from build123d import *

# Parameters (mm, degrees)
EXTRUDE_1_DEPTH     = 360
CUT_EXTRUDE_1_DEPTH = 702.498396292


with BuildPart() as part:
    # 草图1 → 凸台-拉伸1 (new body)
    with BuildSketch(Plane(origin=(0, 0, 0), x_dir=(1, 0, 0), z_dir=(0, 1, 0))):
        Polygon((-225, 0), (225, 0), (225, 250), (100, 400), (-100, 400), (-225, 250), align=None)
    extrude(amount=EXTRUDE_1_DEPTH)

    # 草图2 → 切除-拉伸1 (cut, through all)
    with BuildSketch(Plane(origin=(225, 0, 0), x_dir=(0, 0, -1), z_dir=(1, 0, 0))):
        Polygon((250, 360), (400, 227.712434447), (400, 360), align=None)
    extrude(amount=-CUT_EXTRUDE_1_DEPTH, mode=Mode.SUBTRACT)


solid = part.part
Part model, mm, in its own coordinate system. Give positions to 0.01 mm unless a question says otherwise; leave off trailing zeros. Write each loop counter-clockwise with the first axis right and the second up, starting at its lowest first coordinate (ties: lowest second). Pieces come first, ordered by that corner, then holes.
1) Probe L1, parallel to Z at x = 101, y = 100.5; L2, parallel to Z at x = 22.5, y = 232.5; L3, parallel to Y at x = 62, z = -251. List the from-to ranges inside material, lowest first.
Resolved:
L1: z = -398.8 to 0
L2: z = -394.57 to 0
L3: y = 0 to 359.12
2) Cut at B-B on y = 92. Write the cut outline in (x, z), then the cut area to 3 significant figures.
Resolved:
outline: (-225, -250) - (-100, -400) - (100, -400) - (225, -250) - (225, 0) - (-225, 0) - close
area: 161,000 mm2
3) Cut at A-A on x = 27.5. Write the cut outline in (y, z).
Resolved:
outline: (0, -400) - (227.71, -400) - (360, -250) - (360, 0) - (0, 0) - close
4) Cut at C-C on z = -357. Write the cut outline in (x, y), then the cut area to 3 significant figures.
Resolved:
outline: (-135.83, 0) - (135.83, 0) - (135.83, 265.63) - (-135.83, 265.63) - close
area: 72,200 mm2
5) Pin check, flat tips, straight feed: pin 1 (1 mm diameter, centred on y = 164.5, z = -345.5, fed in from +X); pin 2 (4 mm diameter, centred on y = 284.5, z = -324.5, fed in from -X); pin 3 (1.5 mm diameter, centred on y = 288, z = -264, fed in from -X). Stop position of each tip, or through.
Resolved:
pin 1: stops at x = 145.83
pin 2: stops at x = -164.58
pin 3: stops at x = -213.96
6) Cut at D-D on x = 132. Write the cut outline in (y, z).
Resolved:
outline: (0, -361.6) - (261.58, -361.6) - (360, -250) - (360, 0) - (0, 0) - close
